Read the model definition and answer for the solid it produces. Units are mm, in the model's axes. Give positions to 0.01 mm unless a question says otherwise; leave off trailing zeros. Write each loop counter-clockwise with the first axis right and the second up, starting at its lowest first coordinate (ties: lowest second). Pieces come first, ordered by that corner, then holes. Notation, with made-up numbers: M 56,-26 L 91,-26 A32 cw 91,9 Z; hole C -29.75,4 d4. An arc over 180 degrees is marked long. Put each result on its own line as item: value.
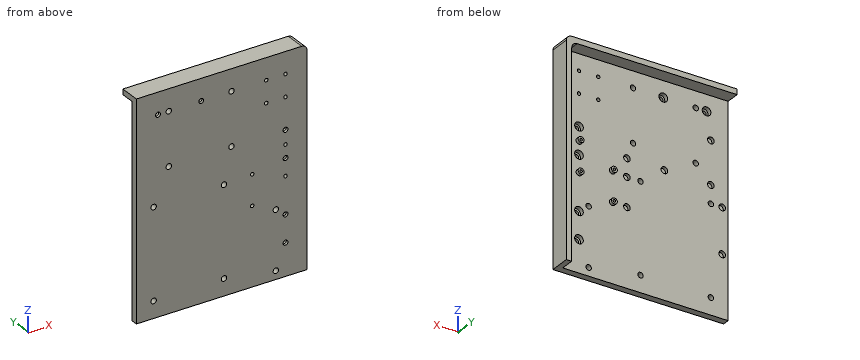
from build123d import *

# Parameters (mm, degrees)
SKETCH1_W                      = 158
SKETCH1_H                      = 199.5
BOSS_EXTRUDE1_DEPTH            = 6.35
BOSS_EXTRUDE2_DEPTH            = 12.7
CBORE_FOR_M4_SHCS1_D           = 4.5
CBORE_FOR_M4_SHCS1_DEPTH       = 6.35
CBORE_FOR_M4_SHCS1_CBORE_D     = 8
CBORE_FOR_M4_SHCS1_CBORE_DEPTH = 4
FILLET2_R                      = 5
FILLET3_R                      = 5
SKETCH8_R                      = 2.5
ESTOP_DEPTH                    = 7.35
SKETCH9_R                      = 2.5
NUCLEOANDPI_DEPTH              = 7.35
SKETCH10_R                     = 2.7
SKETCH10_R_2                   = 1.2
BUCKS_EXTRUDE_DEPTH            = 3
SKETCH11_R                     = 1.6
BUCKS_CUT_DEPTH                = 6.35
BUCK_2_COUNT                   = 2
BUCK_2_PITCH                   = 28
SKETCH12_R                     = 2.5
PI_2_DEPTH                     = 7.35
SKETCH13_R                     = 1.6
IMU_DEPTH                      = 7.35
SKETCH15_R                     = 3.05
MAGNETS_DEPTH                  = 3.1


with BuildPart() as part:
    # Sketch1 → Boss-Extrude1 (new body)
    with BuildSketch(Plane(origin=(0, 0, 0), x_dir=(1, 0, 0), z_dir=(0, 1, 0))):
        with Locations((79, -99.75)):
            Rectangle(SKETCH1_W, SKETCH1_H)
    extrude(amount=BOSS_EXTRUDE1_DEPTH)

    # Sketch3 → Boss-Extrude2 (add)
    with BuildSketch(Plane(origin=(0, 6.35, 0), x_dir=(1, 0, 0), z_dir=(0, 1, 0))):
        Polygon((158, -199.5), (158, 0), (153, 0), (153, -194.5), (0, -194.5), (0, -199.5), align=None)
    extrude(amount=BOSS_EXTRUDE2_DEPTH)

    # CBORE for M4 SHCS1
    with Locations(Plane(origin=(0, 6.35, 0), x_dir=(1, 0, 0), z_dir=(0, 1, 0))):
        with Locations((138, -55), (20, -179.5), (60, -179.5), (138, -130), (138, -105), (138, -30)):
            CounterBoreHole(CBORE_FOR_M4_SHCS1_D / 2, CBORE_FOR_M4_SHCS1_CBORE_D / 2, CBORE_FOR_M4_SHCS1_CBORE_DEPTH, depth=CBORE_FOR_M4_SHCS1_DEPTH)

    # Fillet2
    fillet2_edges = [part.edges().sort_by_distance(p)[0] for p in [
        (158, 9.525, 199.5),
    ]]
    fillet(fillet2_edges, radius=FILLET2_R)

    # Fillet3
    fillet3_edges = [part.edges().sort_by_distance(p)[0] for p in [
        (153, 12.7, 194.5),
    ]]
    fillet(fillet3_edges, radius=FILLET3_R)

    # Sketch8 → eStop (cut, through all)
    with BuildSketch(Plane(origin=(0, 6.35, 0), x_dir=(1, 0, 0), z_dir=(0, 1, 0))):
        with Locations((129.05, -62)):
            Circle(SKETCH8_R)
        with Locations((129.05, -7.75)):
            Circle(SKETCH8_R)
    extrude(amount=-ESTOP_DEPTH, mode=Mode.SUBTRACT)

    # Sketch9 → NucleoAndPi (cut, through all)
    with BuildSketch(Plane(origin=(0, 6.35, 0), x_dir=(1, 0, 0), z_dir=(0, 1, 0))):
        with Locations((16, -15.57)):
            Circle(SKETCH9_R)
        with Locations((81.1, -15.57)):
            Circle(SKETCH9_R)
        with Locations((81.1, -98.77)):
            Circle(SKETCH9_R)
        with Locations((16, -98.77)):
            Circle(SKETCH9_R)
    extrude(amount=-NUCLEOANDPI_DEPTH, mode=Mode.SUBTRACT)

    # Sketch10 → Bucks - Extrude (add)
    with BuildSketch(Plane(origin=(0, 6.35, 0), x_dir=(1, 0, 0), z_dir=(0, 1, 0))):
        with Locations((138, -89)):
            Circle(SKETCH10_R)
        with Locations((138, -89)):
            Circle(SKETCH10_R_2, mode=Mode.SUBTRACT)
        with Locations((107.2, -72)):
            Circle(SKETCH10_R)
        with Locations((107.2, -72)):
            Circle(SKETCH10_R_2, mode=Mode.SUBTRACT)
    bucks_extrude = extrude(amount=BUCKS_EXTRUDE_DEPTH)

    # Sketch11 → Bucks - Cut (cut)
    with BuildSketch(Plane(origin=(0, 6.35, 0), x_dir=(1, 0, 0), z_dir=(0, 1, 0))):
        with Locations((138, -89)):
            Circle(SKETCH11_R)
        with Locations((107.2, -72)):
            Circle(SKETCH11_R)
    bucks_cut = extrude(amount=-BUCKS_CUT_DEPTH, mode=Mode.SUBTRACT)

    # Buck 2: Bucks - Extrude, Bucks - Cut ×2
    with Locations(*[(0, 0, i * BUCK_2_PITCH) for i in range(1, BUCK_2_COUNT)]):
        add(bucks_extrude)
        add(bucks_cut, mode=Mode.SUBTRACT)

    # Sketch12 → Pi 2 (cut, through all)
    with BuildSketch(Plane(origin=(0, 6.35, 0), x_dir=(1, 0, 0), z_dir=(0, 1, 0))):
        with Locations((30, -130.5)):
            Circle(SKETCH12_R)
        with Locations((88, -130.5)):
            Circle(SKETCH12_R)
        with Locations((88, -179.5)):
            Circle(SKETCH12_R)
        with Locations((30, -179.5)):
            Circle(SKETCH12_R)
    extrude(amount=-PI_2_DEPTH, mode=Mode.SUBTRACT)

    # Sketch13 → IMU (cut, through all)
    with BuildSketch(Plane(origin=(0, 6.35, 0), x_dir=(1, 0, 0), z_dir=(0, 1, 0))):
        with Locations((120.22, -159.18)):
            Circle(SKETCH13_R)
        with Locations((120.22, -179.5)):
            Circle(SKETCH13_R)
        with Locations((138, -159.18)):
            Circle(SKETCH13_R)
        with Locations((138, -179.5)):
            Circle(SKETCH13_R)
    extrude(amount=-IMU_DEPTH, mode=Mode.SUBTRACT)

    # Sketch15 → MAGNETS (cut)
    with BuildSketch(Plane(origin=(0, 6.35, 0), x_dir=(1, 0, 0), z_dir=(0, 1, 0))):
        with Locations((5.5, -57.17)):
            Circle(SKETCH15_R)
        with Locations((5.5, -98.77)):
            Circle(SKETCH15_R)
        with Locations((16, -115.385)):
            Circle(SKETCH15_R)
        with Locations((59, -115.385)):
            Circle(SKETCH15_R)
        with Locations((93.65, -98.77)):
            Circle(SKETCH15_R)
        with Locations((93.65, -115.385)):
            Circle(SKETCH15_R)
        with Locations((93.65, -72)):
            Circle(SKETCH15_R)
        with Locations((16, -155)):
            Circle(SKETCH15_R)
    extrude(amount=-MAGNETS_DEPTH, mode=Mode.SUBTRACT)


solid = part.part
(1) Section B-B on z = 105 is taken. Determine the outline of the cut face in (x, y).
Result:
outline: M 0,0 L 135.75,0 L 135.75,2.35 L 134,2.35 L 134,6.35 L 0,6.35 Z; M 140.25,0 L 158,0 L 158,19.05 L 153,19.05 L 153,6.35 L 142,6.35 L 142,2.35 L 140.25,2.35 Z
(2) Section C-C on y = 11.5 is taken. Determine the outline of the cut face in (x, z).
Result:
outline: M 0,194.5 L 148,194.5 A5 cw 153,189.5 L 153,0 L 158,0 L 158,194.5 A5 ccw 153,199.5 L 0,199.5 Z
(3) Section A-A on x = 88 is taken. Determine the outline of the cut face in (y, z).
Result:
outline: M 0,0 L 6.35,0 L 6.35,128 L 0,128 Z; M 0,133 L 6.35,133 L 6.35,177 L 0,177 Z; M 0,182 L 6.35,182 L 6.35,194.5 L 19.05,194.5 L 19.05,199.5 L 0,199.5 Z
(4) Section D-D on x = 38 is taken. Determine the outline of the cut face in (y, z), and give its area (3 significant figures).
Result:
outline: M 0,0 L 6.35,0 L 6.35,194.5 L 19.05,194.5 L 19.05,199.5 L 0,199.5 Z
area: 1,330 mm²
(5) Straight lines are drawn through the part: line 1 along X through (y, z) = (7.7, 100); line 2 along Z through (x, y) = (5.5, 5.1); line 3 along Z through (x, y) = (129.05, 1.75). For each, find the intervals that lie inside material, in ascending order. Write a range as from..to.
Result:
line 1: x = 104.5..106, 108.4..109.9, 153..158
line 2: z = 0..54.12, 60.22..95.72, 101.82..199.5
line 3: z = 0..5.25, 10.25..59.5, 64.5..199.5
(6) Given pin 1 Ø6.5 at (x, z) = (129.05, 62) entering from +Y; pin 2 Ø3.5 at (x, z) = (93.65, 72) entering from +Y; pin 3 Ø1.6 at (x, z) = (106.5, 71.5) entering from +Y; pin 4 Ø1.6 at (x, z) = (107, 72) entering from -Y, each flat-ended and moving along its own axis, determine where each tip first touches the part or whether it passes through.
Result:
pin 1: stops at y = 6.35
pin 2: stops at y = 3.25
pin 3: stops at y = 9.35
pin 4: passes through
